```python
from build123d import *

# Parameters (mm, degrees)
SKETCH1_W                        = 50
SKETCH1_H                        = 100
BOSS_EXTRUDE1_DEPTH              = 25
FILLET1_R                        = 5
SKETCH2_W                        = 25
SKETCH2_H                        = 75
CUT_EXTRUDE1_DEPTH               = 50
FILLET2_R                        = 5
SKETCH4_W                        = 35
SKETCH4_H                        = 35
BOSS_EXTRUDE2_DEPTH              = 15
FILLET7_R                        = 2
FILLET8_R                        = 2
F_10_0MM_DOWEL_HOLE1_D           = 10
F_10_0MM_DOWEL_HOLE1_CSINK_D     = 10.05
F_10_0MM_DOWEL_HOLE1_CSINK_ANGLE = 90


with BuildPart() as part:
    # Sketch1 → Boss-Extrude1 (new, symmetric)
    with BuildSketch(Plane(origin=(0, 0, 0), x_dir=(0, 0, -1), z_dir=(1, 0, 0))):
        Rectangle(SKETCH1_W, SKETCH1_H)
    extrude(amount=BOSS_EXTRUDE1_DEPTH, both=True)

    # Fillet1
    fillet1_edges = [part.edges().sort_by_distance(p)[0] for p in [
        (25, -50, 0),
        (-25, -50, 0),
        (-25, 50, 0),
        (25, 50, 0),
    ]]
    fillet(fillet1_edges, radius=FILLET1_R)

    # Sketch2 → Cut-Extrude1 (cut)
    with BuildSketch(Plane.XY.offset(25)):
        Rectangle(SKETCH2_W, SKETCH2_H)
    extrude(amount=-CUT_EXTRUDE1_DEPTH, mode=Mode.SUBTRACT)

    # Fillet2
    fillet2_edges = [part.edges().sort_by_distance(p)[0] for p in [
        (12.5, 37.5, 0),
        (12.5, -37.5, 0),
        (-12.5, -37.5, 0),
        (-12.5, 37.5, 0),
    ]]
    fillet(fillet2_edges, radius=FILLET2_R)

    # Sketch4 → Boss-Extrude2 (add)
    with BuildSketch(Plane.ZY.offset(25)):
        Rectangle(SKETCH4_W, SKETCH4_H)
    boss_extrude2 = extrude(amount=BOSS_EXTRUDE2_DEPTH)

    # Mirror1: Boss-Extrude2 across plane
    add(boss_extrude2.mirror(Plane(origin=(0, 0, 0), x_dir=(0, 0, 1), z_dir=(1, 0, 0))))

    # Sketch6 → Revolve1 (revolve)
    with BuildSketch(Plane.XY, mode=Mode.PRIVATE) as revolve1_sk:
        Polygon((-40, 15), (-43, 15), (-43, 9), (-45, 9), (-45, 11), (-65, 11), (-65, 0), (-40, 0), align=None)
    revolve1 = revolve(revolve1_sk.sketch.rotate(Axis((0, 0, 0), (-1, 0, 0)), 90), axis=Axis((0, 0, 0), (-1, 0, 0)))

    # Mirror2: Revolve1 across plane
    add(revolve1.mirror(Plane(origin=(0, 0, 0), x_dir=(0, 0, 1), z_dir=(1, 0, 0))))

    # Fillet7
    fillet7_edges = [part.edges().sort_by_distance(p)[0] for p in [
        (-65, 0, 11),
    ]]
    fillet(fillet7_edges, radius=FILLET7_R)

    # Fillet8
    fillet8_edges = [part.edges().sort_by_distance(p)[0] for p in [
        (65, 0, 11),
    ]]
    fillet(fillet8_edges, radius=FILLET8_R)

    # Ø10.0mm Dowel Hole1 (through all)
    with Locations(Plane.XY.offset(25)):
        with Locations((18.5, 25), (18.5, -25), (-18.5, -25), (-18.5, 25)):
            CounterSinkHole(F_10_0MM_DOWEL_HOLE1_D / 2, F_10_0MM_DOWEL_HOLE1_CSINK_D / 2, counter_sink_angle=F_10_0MM_DOWEL_HOLE1_CSINK_ANGLE)


solid = part.part
```
The listing builds one solid part. Answer for the finished solid, in the listing's coordinates (mm). A direction names the side the tool comes from. Give positions to 0.01 mm unless a question says otherwise; leave off trailing zeros. Write each loop counter-clockwise with the first axis right and the second up, starting at its lowest first coordinate (ties: lowest second). Pieces come first, ordered by that corner, then holes. Notation, with made-up numbers: (79, 19) -> (127, 19) arc R23 ccw to (127, 53) -> close; hole circle Ø1 at (-13.75, 2.25). An arc over 180 degrees is marked (long way). Write item = value, one per line. Start each with the question number.
1) The part is cut by section A-A, the plane x = 3. Determine the outline of the cut face in (y, z).
2) Each of these flat-tipped pins is pushed along its axis until it touches: pin 1 (4.5 mm diameter, centred on x = -29.5, z = 4.5, fed in from -Y); pin 2 (7.5 mm diameter, centred on x = 34.5, z = 8, fed in from +Y); pin 3 (12 mm diameter, centred on x = 29, z = 0, fed in from -Y). Where does it stop, or does it pass through?
3) Determine the mould class of faces 4 (the face through (65, 0, 0)), 5 (the face through (24, 48, 0)), 6 (the face through (19.58, -29.88, -0.36)) for opening direction Y: +Y half, -Y half, draft (parallel to the pull), parting line (faces both ways), or undercut.
4) Straight lines are drawn through the part: line 1 along Y through (x, z) = (18.5, -11); line 2 along X through (y, z) = (-25, 0); line 3 along Y through (x, z) = (-1, 18.5). For each, find the intervals that lie inside material, in ascending order.
5) The part is cut by section D-D, the plane y = -42. Determine the outline of the cut face in (x, z).
6) The part is cut by section B-B, the plane y = 25. Determine the outline of the cut face in (x, z) (3 decimals), and give its area (3 significant figures).
7) The part is cut by section C-C, the plane z = 0. Count the separate pieces of the cut face and the enclosed holes in it, and give its area (3 significant figures).
8) Which of the six approach directions +Z, -Z, +X, -X, +Y, -Y give full straight-line access (tool end or side, diameter ignored) to faces 1 (the face through (32, 0, 17.5)), 2 (the face through (11, 36.07, -0.35)), 3 (the face through (45, 9, 2))?
Solutions:
q1.outline = (-50, -25) -> (-37.5, -25) -> (-37.5, 25) -> (-50, 25) -> close; (37.5, -25) -> (50, -25) -> (50, 25) -> (37.5, 25) -> close
q2.pin_1 = -17.5
q2.pin_2 = 17.5
q2.pin_3 = -49
q3.face_4 = draft
q3.face_5 = +Y half
q3.face_6 = undercut
q4.line_1 = -50 to -30, -20 to 20, 30 to 50
q4.line_2 = -25 to -23.5, -13.5 to -12.5, 12.5 to 13.5, 23.5 to 25
q4.line_3 = -50 to -37.5, 37.5 to 50
q5.outline = (-25, -25) -> (25, -25) -> (25, 25) -> (-25, 25) -> close
q6.outline = (-25, -25) -> (-23.5, -25) -> (-23.5, 24.975) -> (-23.525, 25) -> (-25, 25) -> close; (-13.5, -25) -> (-12.5, -25) -> (-12.5, 25) -> (-13.475, 25) -> (-13.5, 24.975) -> close; (12.5, -25) -> (13.5, -25) -> (13.5, 24.975) -> (13.475, 25) -> (12.5, 25) -> close; (23.5, -25) -> (25, -25) -> (25, 25) -> (23.525, 25) -> (23.5, 24.975) -> close
q6.area = 250 mm²
q7.separate_pieces = 1
q7.enclosed_holes = 5
q7.area = 4,990 mm²
q8.face_1 = +Z, +X, +Y, -Y
q8.face_2 = +Z, -Z
q8.face_3 = none
